Autodesk Inventor part; units mm, degrees
ref_plane "YZ Plane" through (0, 0, 0) normal (1, 0, 0) x (0, 1, 0)
ref_plane "XZ Plane" through (0, 0, 0) normal (0, 1, 0) x (-1, 0, 0)
ref_plane "XY Plane" through (0, 0, 0) normal (0, 0, 1) x (1, 0, 0)
sketch "Sketch1" plane through (0, 0, 0) normal (0, 0, 1) x (1, 0, 0)
  circle A0 centre (0, 0) radius 7.5
  circle A1 centre (0, 0) radius 2.75
  dimension "d0" = 15
  dimension "d1" = 5.5
extrude "Extrusion1" add sketch "Sketch1" along normal blind 5
sketch "Sketch2" plane through (0, 0, 5) normal (0, 0, 1) x (1, 0, 0)
  circle A0 centre (0, 0) radius 15
  arc A1 (18.8661, 0.9) -> (14.8661, 2) centre (12.9269, -12.8741) ccw
  arc A2 (18.8661, -0.9) -> (18.8661, 0.9) centre (-1.1137, 0) ccw
  line L0 (0, 0) -> (23.4972, 0) construction
  arc A3 (14.8661, -2) -> (18.8661, -0.9) centre (12.9269, 12.8741) ccw
  arc A4 (14.8661, -2) -> (14.8661, 2) centre (0, 0) ccw
  arc A5 (17.5516, 6.977) -> (13.4112, 6.7186) centre (16.4067, -7.9792) ccw
  arc A6 (18.1361, 5.2746) -> (17.5516, 6.977) centre (-1.0533, -0.3616) ccw
  arc A7 (14.71, 2.9354) -> (18.1361, 5.2746) centre (8.0463, 16.3739) ccw
  arc A8 (14.71, 2.9354) -> (13.4112, 6.7186) centre (0, 0) ccw
  arc A9 (14.3352, 12.298) -> (10.503, 10.7092) centre (18.1086, -2.2196) ccw
  arc A10 (15.4408, 10.8776) -> (14.3352, 12.298) centre (-0.8788, -0.684) ccw
  arc A11 (12.9598, 7.5526) -> (15.4408, 10.8776) centre (2.2937, 18.0994) ccw
  arc A12 (12.9598, 7.5526) -> (10.503, 10.7092) centre (0, 0) ccw
  arc A13 (9.5653, 16.2863) -> (6.4566, 13.5393) centre (17.8482, 3.7805) ccw
  arc A14 (11.0722, 15.3018) -> (9.5653, 16.2863) centre (-0.6091, -0.9323) ccw
  arc A15 (9.8053, 11.3515) -> (11.0722, 15.3018) centre (-3.7074, 17.8635) ccw
  arc A16 (9.8053, 11.3515) -> (6.4566, 13.5393) centre (0, 0) ccw
  arc A17 (3.7589, 18.5097) -> (1.7106, 14.9021) centre (15.6536, 9.371) ccw
  arc A18 (5.5038, 18.0678) -> (3.7589, 18.5097) centre (-0.2734, -1.0796) ccw
  arc A19 (5.5882, 13.9202) -> (5.5038, 18.0678) centre (-9.3068, 15.6918) ccw
  arc A20 (5.5882, 13.9202) -> (1.7106, 14.9021) centre (0, 0) ccw
  arc A21 (-2.4549, 18.7273) -> (-3.2208, 14.6501) centre (11.7627, 13.9459) ccw
  arc A22 (-0.661, 18.876) -> (-2.4549, 18.7273) centre (0.092, -1.1099) ccw
  arc A23 (0.7655, 14.9805) -> (-0.661, 18.876) centre (-13.8977, 11.8196) ccw
  arc A24 (0.7655, 14.9805) -> (-3.2208, 14.6501) centre (0, 0) ccw
  arc A25 (-8.4026, 16.9155) -> (-7.8032, 12.8106) centre (6.5971, 17.0096) ccw
  arc A26 (-6.7542, 17.6386) -> (-8.4026, 16.9155) centre (0.4474, -1.0199) ccw
  arc A27 (-4.1401, 14.4173) -> (-6.7542, 17.6386) centre (-16.9825, 6.6667) ccw
  arc A28 (-4.1401, 14.4173) -> (-7.8032, 12.8106) centre (0, 0) ccw
  arc A29 (-13.4398, 13.2707) -> (-11.54, 9.5828) centre (0.7166, 18.2301) ccw
  arc A30 (-12.1155, 14.4898) -> (-13.4398, 13.2707) centre (0.7543, -0.8194) ccw
  arc A31 (-8.5971, 12.2919) -> (-12.1155, 14.4898) centre (-18.227, 0.7912) ccw
  arc A32 (-8.5971, 12.2919) -> (-11.54, 9.5828) centre (0, 0) ccw
  arc A33 (-17.0206, 8.1877) -> (-14.0262, 5.3165) centre (-5.2415, 17.475) ccw
  arc A34 (-16.1639, 9.7708) -> (-17.0206, 8.1877) centre (0.9794, -0.53) ccw
  arc A35 (-12.1224, 8.8344) -> (-16.1639, 9.7708) centre (-17.4963, -5.1699) ccw
  arc A36 (-12.1224, 8.8344) -> (-14.0262, 5.3165) centre (0, 0) ccw
  arc A37 (-18.7569, 2.2175) -> (-14.9925, 0.4742) centre (-10.6316, 14.8262) ccw
  arc A38 (-18.4606, 3.993) -> (-18.7569, 2.2175) centre (1.0985, -0.1833) ccw
  arc A39 (-14.3341, 4.4196) -> (-18.4606, 3.993) centre (-14.8696, -10.5708) ccw
  arc A40 (-14.3341, 4.4196) -> (-14.9925, 0.4742) centre (0, 0) ccw
  arc A41 (-18.4606, -3.993) -> (-14.3341, -4.4196) centre (-14.8696, 10.5708) ccw
  arc A42 (-18.7569, -2.2175) -> (-18.4606, -3.993) centre (1.0985, 0.1833) ccw
  arc A43 (-14.9925, -0.4742) -> (-18.7569, -2.2175) centre (-10.6316, -14.8262) ccw
  arc A44 (-14.9925, -0.4742) -> (-14.3341, -4.4196) centre (0, 0) ccw
  arc A45 (-16.1639, -9.7708) -> (-12.1224, -8.8344) centre (-17.4963, 5.1699) ccw
  arc A46 (-17.0206, -8.1877) -> (-16.1639, -9.7708) centre (0.9794, 0.53) ccw
  arc A47 (-14.0262, -5.3165) -> (-17.0206, -8.1877) centre (-5.2415, -17.475) ccw
  arc A48 (-14.0262, -5.3165) -> (-12.1224, -8.8344) centre (0, 0) ccw
  arc A49 (-12.1155, -14.4898) -> (-8.5971, -12.2919) centre (-18.227, -0.7912) ccw
  arc A50 (-13.4398, -13.2707) -> (-12.1155, -14.4898) centre (0.7543, 0.8194) ccw
  arc A51 (-11.54, -9.5828) -> (-13.4398, -13.2707) centre (0.7166, -18.2301) ccw
  arc A52 (-11.54, -9.5828) -> (-8.5971, -12.2919) centre (0, 0) ccw
  arc A53 (-6.7542, -17.6386) -> (-4.1401, -14.4173) centre (-16.9825, -6.6667) ccw
  arc A54 (-8.4026, -16.9155) -> (-6.7542, -17.6386) centre (0.4474, 1.0199) ccw
  arc A55 (-7.8032, -12.8106) -> (-8.4026, -16.9155) centre (6.5971, -17.0096) ccw
  arc A56 (-7.8032, -12.8106) -> (-4.1401, -14.4173) centre (0, 0) ccw
  arc A57 (-0.661, -18.876) -> (0.7655, -14.9805) centre (-13.8977, -11.8196) ccw
  arc A58 (-2.4549, -18.7273) -> (-0.661, -18.876) centre (0.092, 1.1099) ccw
  arc A59 (-3.2208, -14.6501) -> (-2.4549, -18.7273) centre (11.7627, -13.9459) ccw
  arc A60 (-3.2208, -14.6501) -> (0.7655, -14.9805) centre (0, 0) ccw
  arc A61 (5.5038, -18.0678) -> (5.5882, -13.9202) centre (-9.3068, -15.6918) ccw
  arc A62 (3.7589, -18.5097) -> (5.5038, -18.0678) centre (-0.2734, 1.0796) ccw
  arc A63 (1.7106, -14.9021) -> (3.7589, -18.5097) centre (15.6536, -9.371) ccw
  arc A64 (1.7106, -14.9021) -> (5.5882, -13.9202) centre (0, 0) ccw
  arc A65 (11.0722, -15.3018) -> (9.8053, -11.3515) centre (-3.7074, -17.8635) ccw
  arc A66 (9.5653, -16.2863) -> (11.0722, -15.3018) centre (-0.6091, 0.9323) ccw
  arc A67 (6.4566, -13.5393) -> (9.5653, -16.2863) centre (17.8482, -3.7805) ccw
  arc A68 (6.4566, -13.5393) -> (9.8053, -11.3515) centre (0, 0) ccw
  arc A69 (15.4408, -10.8776) -> (12.9598, -7.5526) centre (2.2937, -18.0994) ccw
  arc A70 (14.3352, -12.298) -> (15.4408, -10.8776) centre (-0.8788, 0.684) ccw
  arc A71 (10.503, -10.7092) -> (14.3352, -12.298) centre (18.1086, 2.2196) ccw
  arc A72 (10.503, -10.7092) -> (12.9598, -7.5526) centre (0, 0) ccw
  arc A73 (18.1361, -5.2746) -> (14.71, -2.9354) centre (8.0463, -16.3739) ccw
  arc A74 (17.5516, -6.977) -> (18.1361, -5.2746) centre (-1.0533, 0.3616) ccw
  arc A75 (13.4112, -6.7186) -> (17.5516, -6.977) centre (16.4067, 7.9792) ccw
  arc A76 (13.4112, -6.7186) -> (14.71, -2.9354) centre (0, 0) ccw
  circle A77 centre (0, 0) radius 2.75
  point P0 (18.8863, 0)
  point P1 (17.863, 6.1324)
  point P2 (14.904, 11.6002)
  point P3 (10.3298, 15.811)
  point P4 (4.6363, 18.3084)
  point P5 (-1.5596, 18.8218)
  point P6 (-7.5866, 17.2956)
  point P7 (-12.7914, 13.8951)
  point P8 (-16.61, 8.9889)
  point P9 (-18.6287, 3.1086)
  point P10 (-18.6287, -3.1086)
  point P11 (-16.61, -8.9889)
  point P12 (-12.7914, -13.8951)
  point P13 (-7.5866, -17.2956)
  point P14 (-1.5596, -18.8218)
  point P15 (4.6363, -18.3084)
  point P16 (10.3298, -15.811)
  point P17 (14.904, -11.6002)
  point P18 (17.863, -6.1324)
  dimension "d4" = 30
  dimension "d5" = 15
  dimension "d6" = 4
  dimension "d7" = 1.8
  dimension "d8" = 20
  dimension "d10" = 2
  dimension "d11" = 15
  dimension "d12" = 4
  dimension "d13" = 2
  dimension "d16" = 360
extrude "Extrusion2" add sketch "Sketch2" along normal blind 10 contours A0 | A0 A1 A2 A3 | A0 A5 A6 A7 | A73 A74 A75 A0 | A0 A9 A10 A11 | A69 A70 A71 A0 | A0 A13 A14 A15 | A65 A66 A67 A0 | A0 A17 A18 A19 | A61 A62 A63 A0 | A0 A21 A22 A23 | A57 A58 A59 A0 | A0 A25 A26 A27 | A53 A54 A55 A0 | A0 A29 A30 A31 | A49 A50 A51 A0 | A0 A33 A34 A35 | A45 A46 A47 A0 | A0 A37 A38 A39 | A41 A42 A43 A0 | A77
sketch "Sketch3" plane through (0, 0, 15) normal (0, 0, 1) x (1, 0, 0)
  circle A0 centre (0, 0) radius 2.75
  dimension "d22" = 5.5
extrude "Extrusion3" cut sketch "Sketch3" against normal through all
properties part number "BA009" material "ABS Plastic"
Verification items for the finished model (mm, model axes). A direction names the side the tool comes from. Round coordinates to 2 decimals unless told otherwise and drop trailing zeros. Write each loop counter-clockwise with the first axis right and the second up, starting at its lowest first coordinate (ties: lowest second). Pieces come first, ordered by that corner, then holes. Notation, with made-up numbers: (20.25, 45.5) - (74.25, 45.5) arc R29 cw to (74.25, 72.5) - close; hole circle Ø5 at (82.5, 44). An arc over 180 degrees is marked (long way). Answer as a JSON object with one key per item and string values. Group by question number.
Q1. Tool access check on faces 1 (the cylindrical face through (15.502, -6.993, 9.93)), 2 (the cylindrical face through (14.797, -2.462, 9.93)), 3 (the cylindrical face through (2.624, -16.802, 9.93)). Record the directions out of +Z, -Z, +X, -X, +Y, -Y that give a thin tool (end or side, any length) a straight path to the whole face; none if there is none.
Q2. Section check C-C, the plane x = 0. Enter the section's corners in (y, z), plus the area to 3 significant figures.
Q3. Section check A-A, the plane y = 0. Enter the section's corners in (x, z), plus the area to 3 significant figures.
Q4. Go/stop test with flat-tipped pins: pin 1 Ø2 at (x, y) = (-5.5, 5) entering from -Z; pin 2 Ø4 at (x, y) = (-13.5, 6.5) entering from -Z; pin 3 Ø3 at (x, z) = (-7.5, 11) entering from -Y; pin 4 Ø8 at (x, z) = (-15, 4.5) entering from -Y. Record where each tip stops, or that it passes through.
Q5. Section check B-B, the plane x = 16.5. Enter the section's corners in (y, z), plus the area to 3 significant figures.
Q6. Thickness scan on line 1 (X direction, y = -16.5, z = 6.75); line 2 (X direction, y = 16, z = 9); line 3 (Z direction, x = 9.5, y = -2). Record the ranges inside material, lowest first.
Q7. Section check D-D, the plane z = 4.5. Enter the section's corners in (x, y), plus the area to 3 significant figures.
Found:
{
 "1": {"face 1": "+Z, -Z", "face 2": "+Z, -Z, +X", "face 3": "+Z, -Z, -Y"},
 "2": {"outline": "(-17.46, 5) - (-7.5, 5) - (-7.5, 0) - (-2.75, 0) - (-2.75, 15) - (-17.46, 15) - close; (2.75, 0) - (7.5, 0) - (7.5, 5) - (17.46, 5) - (17.46, 15) - (2.75, 15) - close", "area": "342 mm^2"},
 "3": {"outline": "(-15, 5) - (-7.5, 5) - (-7.5, 0) - (-2.75, 0) - (-2.75, 15) - (-15, 15) - close; (2.75, 0) - (7.5, 0) - (7.5, 5) - (18.89, 5) - (18.89, 15) - (2.75, 15) - close", "area": "331 mm^2"},
 "4": {"pin 1": "stops at z = 0", "pin 2": "stops at z = 5", "pin 3": "stops at y = -17.64", "pin 4": "stops at y = -14.49"},
 "5": {"outline": "(-7.02, 5) - (-3.98, 5) - (-3.98, 15) - (-7.02, 15) - close; (-1.69, 5) - (1.69, 5) - (1.69, 15) - (-1.69, 15) - close; (3.98, 5) - (7.02, 5) - (7.02, 15) - (3.98, 15) - close", "area": "94.6 mm^2"},
 "6": {"line 1": "x = -8.39 to -5.66, -3.02 to 0.35, 2.46 to 5.67", "line 2": "x = -8.37 to -5.24, -3.1 to 0.51, 2.2 to 5.69, 9.15 to 10.03", "line 3": "z = 5 to 15"},
 "7": {"outline": "circle Ø15 at (0, 0); hole circle Ø5.5 at (0, 0)", "area": "153 mm^2"}
}
